Could you check a few things on this drawing? It's one solid part, dimensions in mm from its lowest x, y, z. Coordinates: 2 decimals unless noted, no trailing zeros. Answer as a JSON object with one key per item and string values. Group by question number.
1) Please list where these lines run through material, in increasing order: line 1 along X through (y, z) = (6.35, 11); line 2 along Y through (x, z) = (6.5, 17.5) (1 decimal); line 3 along Z through (x, y) = (5.5, 11.75).
2) We'd pull the mould along Y, two halves only. Please class the marked faces 1, 2 and 3: released by +Y, released by -Y, zero draft, split by the parting line, or undercut.
3) Will these pins go through, and if not, where does the flat tip stop? pin 1 Ø0.6 at (x, z) = (1, 3.5) entering from +Y (1 decimal); pin 2 Ø5 at (x, y) = (6.34, 6.35) entering from +Z; pin 3 Ø6 at (y, z) = (9.5, 17.5) entering from +X; pin 4 Ø1 at (y, z) = (10.5, 12.5) entering from -X (1 decimal).
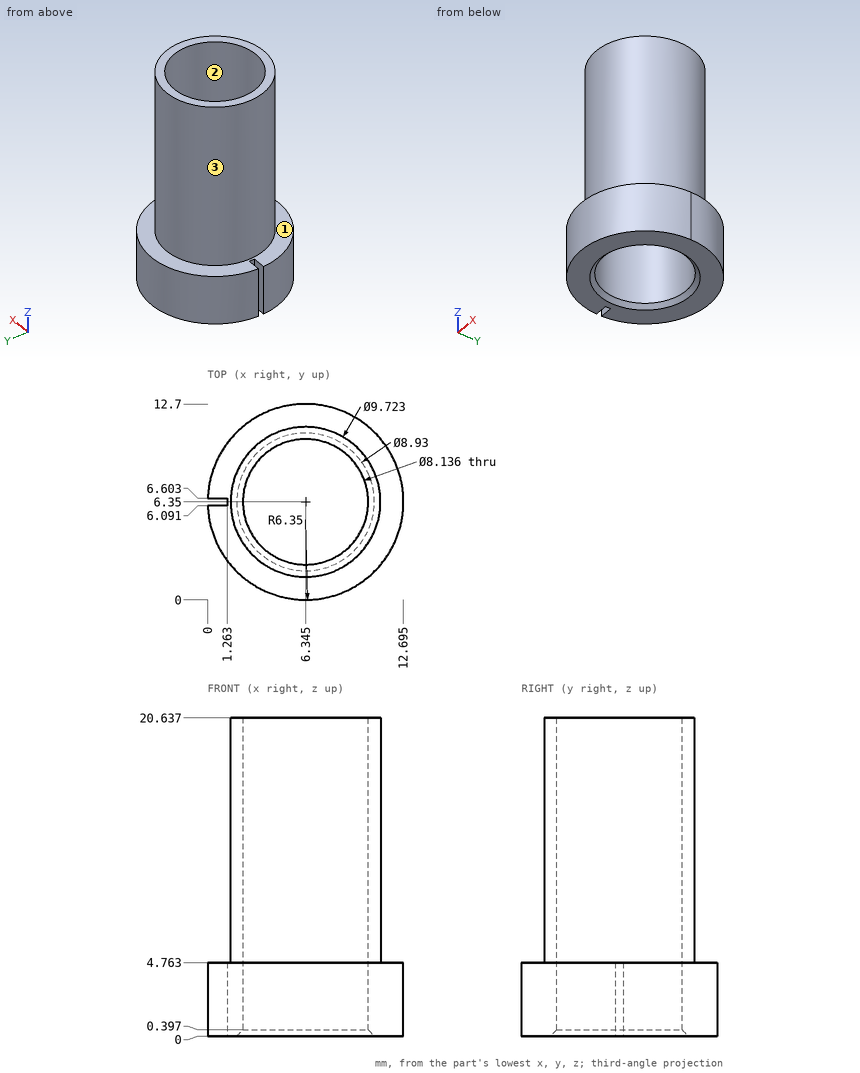
Here are the results:
{
 "1": {"line 1": "x = 1.48 to 2.28, 10.41 to 11.21", "line 2": "y = 1.5 to 2.3, 10.4 to 11.2", "line 3": "z = 0 to 4.76"},
 "2": {"face 1": "zero draft", "face 2": "undercut", "face 3": "split by the parting line"},
 "3": {"pin 1": "stops at y = 10.2", "pin 2": "passes through", "pin 3": "stops at x = 11.2", "pin 4": "stops at x = 3.1"}
}
